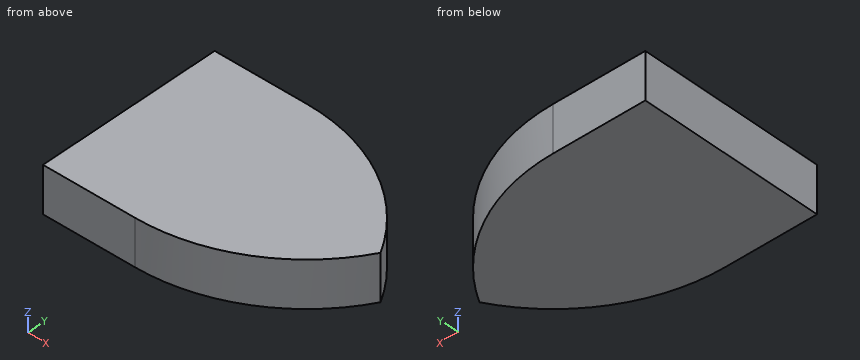
from build123d import *

# Parameters (mm, degrees)
F0_W        = 60
F0_H        = 10
F1_DEPTH    = 40
F2_T1_DEPTH = 210


# Not quite as in the source:
# - a fillet or chamfer that OpenCascade refuses, or shapes differently, is made with other operations: its cross-section is extruded or revolved along the edge and cut away or added


with BuildPart() as f1:
    # F0 (on Front) → F1 (new body)
    with BuildSketch(Plane.XZ):
        with Locations((2.7074571699, -10.2079533711)):
            Rectangle(F0_W, F0_H)
    extrude(amount=F1_DEPTH)

    # F2: fillet of radius 40 on 2 edges, made by hand

    # F2_s2 → F2_t1 (cut)
    with BuildSketch(Plane.XY.offset(-115.2079533711)):
        with BuildLine():
            ThreePointArc((32.7074571699, 0), (20.9917284174, -28.2842712475), (-7.2925428301, -40))
            Line((-7.2925428301, -40), (32.7074571699, -40))
            Line((32.7074571699, -40), (32.7074571699, 0))
        make_face()
        with BuildLine():
            ThreePointArc((32.7074571699, -40), (20.9917284174, -11.7157287525), (-7.2925428301, 0))
            Line((-7.2925428301, 0), (32.7074571699, 0))
            Line((32.7074571699, 0), (32.7074571699, -40))
        make_face()
    extrude(amount=F2_T1_DEPTH, mode=Mode.SUBTRACT)


solid = f1.part
Could you check a few things on this model? Use its own coordinates, in mm. Coordinates: 2 decimals unless noted, no trailing zeros. Order: outer loops, then holes, each group sorted by start corner. A loop starts at its lowest first (then second) coordinate and runs counter-clockwise, first axis right, second up.
Q1. Suppose I cut it at C-C on x = 7.5. Please give me the cut outline in (y, z).
Q2. Please list where these lines run through material, in increasing order: L1, parallel to Y at x = 23.5, z = -9; L2, parallel to X at y = -26.5, z = -7.75; L3, parallel to X at y = -25, z = -13.25.
Q3. Will these pins go through, and if not, where does the flat tip stop? pin 1 (3 mm diameter, centred on x = 13, z = -6.5, fed in from -Y); pin 2 (2 mm diameter, centred on x = -2, z = -11.5, fed in from -Y).
Q4. Suppose I cut it at B-B on y = -13. Please give me the cut outline in (x, z), and give its area (3 significant figures).
Q5. Suppose I cut it at A-A on z = -13. Please give me the cut outline in (x, y), and give its area (3 significant figures).
Answer:
1. outline: (-37.16, -15.21) - (-2.84, -15.21) - (-2.84, -5.21) - (-37.16, -5.21) - close
2. L1: y = -25.53 to -14.47
2. L2: x = -27.29 to 22.67
2. L3: x = -27.29 to 23.93
3. pin 1: stops at y = -35.31
3. pin 2: stops at y = -39.77
4. outline: (-27.29, -15.21) - (22.22, -15.21) - (22.22, -5.21) - (-27.29, -5.21) - close
4. area: 495 mm2
5. outline: (-27.29, -40) - (-7.29, -40) arc R40 ccw to (27.35, -20) arc R40 ccw to (-7.29, 0) - (-27.29, 0) - close
5. area: 1,780 mm2
